Autodesk Inventor part; units mm, degrees
ref_plane "YZ Plane" through (0, 0, 0) normal (1, 0, 0) x (0, 1, 0)
ref_plane "XZ Plane" through (0, 0, 0) normal (0, 1, 0) x (-1, 0, 0)
ref_plane "XY Plane" through (0, 0, 0) normal (0, 0, 1) x (1, 0, 0)
sketch "Sketch1" plane through (0, 0, 0) normal (0, 1, 0) x (-1, 0, 0)
  line L0 (0, 0) -> (40.5, 0)
  line L1 (40.5, 0) -> (40.5, -20)
  line L2 (40.5, -20) -> (0, -20)
  line L3 (0, -20) -> (0, 0)
  dimension "d0" = 20
  dimension "d1" = 40.5
extrude "Extrusion1" add sketch "Sketch1" along normal blind 28
sketch "Sketch2" plane through (0, 28, 0) normal (0, 1, 0) x (1, 0, 0)
  line L0 (7.25, 0) -> (-47.75, 0)
  line L1 (-47.75, 0) -> (-47.75, 20)
  line L2 (-47.75, 20) -> (7.25, 20)
  line L3 (7.25, 20) -> (7.25, 0)
  line L4 (0, 20) -> (-40.5, 20)
  line L5 (-40.5, 20) -> (-40.5, 0)
  line L6 (-40.5, 0) -> (0, 0)
  dimension "d4" = 0
  dimension "d5" = 55
  dimension "d6" = 7.25
  dimension "d7" = 0
extrude "Extrusion2" add sketch "Sketch2" along normal blind 3.5
sketch "Sketch3" plane through (0, 31.5, 0) normal (0, 1, 0) x (1, 0, 0)
  circle A0 centre (-44.75, 5) radius 2.5
  circle A1 centre (-44.75, 15) radius 2.5
  line L0 (-47.75, 0) -> (7.25, 0)
  line L1 (7.25, 20) -> (-47.75, 20)
  line L2 (-47.75, 20) -> (-47.75, 0)
  point P0 (0, 0)
  dimension "d10" = 5
  dimension "d11" = 5
  dimension "d12" = 5
  dimension "d14" = 5
  dimension "d15" = 3
  dimension "d16" = 3
extrude "Extrusion3" cut sketch "Sketch3" against normal blind 3.5
ref_plane "Work Plane1" through (-20.25, 28, 0) normal (1, 0, 0) x (0, 0, -1)
mirror "Mirror1" about plane through (-20.25, 28, 0) normal (1, 0, 0) of "Extrusion3"
sketch "Sketch4" plane through (0, 31.5, 0) normal (0, 1, 0) x (1, 0, 0)
  line L0 (0, 0) -> (-40.5, 0)
  line L1 (-40.5, 0) -> (-40.5, 20)
  line L2 (-40.5, 20) -> (0, 20)
  line L3 (0, 20) -> (0, 0)
extrude "Extrusion4" add sketch "Sketch4" along normal blind 10
sketch "Sketch5" plane through (0, 41.5, 0) normal (0, 1, 0) x (1, 0, 0)
  circle A0 centre (-9, 10) radius 2.75
  line L0 (0, 0) -> (0, 20)
  line L1 (-40.5, 0) -> (0, 0)
  line L2 (-40.5, 20) -> (-40.5, 0)
  dimension "d22" = 10
  dimension "d23" = 5.5
  dimension "d40" = 31.5
extrude "Extrusion5" add sketch "Sketch5" along normal blind 6.5
sketch "Sketch6" plane through (0, 0, 0) normal (1, 0, 0) x (0, 0, -1)
  line L0 (6.75, 3) -> (13.25, 3)
  line L1 (13.25, 3) -> (13.25, 6.5)
  line L2 (13.25, 6.5) -> (6.75, 6.5)
  line L3 (6.75, 6.5) -> (6.75, 3)
  line L4 (0, 0) -> (20, 0)
  line L5 (0, 0) -> (0, 28)
  dimension "d26" = 3
  dimension "d27" = 6.5
  dimension "d28" = 3.5
  dimension "d29" = 6.75
extrude "Extrusion6" add sketch "Sketch6" along normal blind 6
sketch "Sketch7" plane through (6, 0, 0) normal (1, 0, 0) x (0, 0, -1)
  circle A0 centre (11.75, 4.75) radius 1.5
  circle A1 centre (8.25, 4.75) radius 1.5
  line L0 (6.75, 6.5) -> (6.75, 3)
  line L1 (13.25, 3) -> (13.25, 6.5)
  line L2 (6.75, 3) -> (13.25, 3)
  point P0 (0, 0)
  dimension "d32" = 3
  dimension "d33" = 3
  dimension "d34" = 1.5
  dimension "d35" = 1.5
  dimension "d36" = 1.75
  dimension "d37" = 1.75
extrude "Extrusion7" add sketch "Sketch7" along normal blind 30
equation "\"d33\" = d32"
equation "\"d37\" = d36"
properties part number "motor_25kg"
Input: part model. Units: mm. Frame: model coordinates. A direction names the side the tool comes from. Give positions to 0.01 mm unless a question says otherwise; leave off trailing zeros. Write each loop counter-clockwise with the first axis right and the second up, starting at its lowest first coordinate (ties: lowest second). Pieces come first, ordered by that corner, then holes. Notation, with made-up numbers: (-16.5, -15.75) -> (32.5, -15.75) arc R5 ccw to (32.5, -10.75) -> close; hole circle Ø9 at (-5.5, -2). An arc over 180 degrees is marked (long way). Use one line per item in the form item = value. Start each with the question number.
1) Ray query, probe 1 along X at (y, z) = (29, -15); probe 2 along Z at (x, y) = (4, 29); probe 3 along X at (y, z) = (7, -8.5). Return the intervals inside material, ascending. Write a range as from..to.
2) Section query B-B on z = -5. Return the cut outline in (x, y), then the cut area to 3 significant figures.
3) Draft query along Z for faces 4 (the flat face through (6, 5, -10)), 5 (the flat face through (-21, 20, -20)), 6 (the cylindrical face through (-6.46, 44.7, -11.05)). Return one class per face: pulls with the +Z half, pulls with the -Z half, needs draft (parallel to the pull), parting line crosses it, or undercut.
4) Section query C-C on y = 30. Return the cut outline in (x, z), then the cut area to 3 significant figures.
5) Pin query (flat end, axial travel): pin 1 (3 mm diameter, centred on x = 2, z = -8.5, fed in from -Y); pin 2 (5 mm diameter, centred on y = 12, z = -12.5, fed in from -X); pin 3 (1.8 mm diameter, centred on y = 30, z = -8, fed in from +X); pin 4 (3 mm diameter, centred on x = 4.25, z = -5, fed in from -Y). Return the tip coordinate at first contact, or that it passes through.
6) Section query D-D on x = -9. Return the cut outline in (y, z).
7) Set-up query: faces 1 (the flat face through (3, 3, -10)), 2 (the cylindrical face through (1.865, 29.774, -4.249)), 3 (the flat face through (3, 5, -13.25)). Return all of +Z, -Z, +X, -X, +Y, -Y with unobstructed straight access to the full face (end or side cutting, diameter ignored); none if empty.
8) Section query A-A on x = 4.25. Return the cut outline in (y, z).
Outcome:
q1.probe_1 = -47.75..-47.25, -42.25..1.75, 6.75..7.25
q1.probe_2 = -20..-17.49, -12.51..-7.49, -2.51..0
q1.probe_3 = -40.5..0
q2.outline = (-47.75, 28) -> (-47.25, 28) -> (-47.25, 31.5) -> (-47.75, 31.5) -> close; (-42.25, 28) -> (-40.5, 28) -> (-40.5, 0) -> (0, 0) -> (0, 28) -> (1.75, 28) -> (1.75, 31.5) -> (0, 31.5) -> (0, 41.5) -> (-40.5, 41.5) -> (-40.5, 31.5) -> (-42.25, 31.5) -> close; (6.75, 28) -> (7.25, 28) -> (7.25, 31.5) -> (6.75, 31.5) -> close
q2.area = 1,700 mm^2
q3.face_4 = undercut
q3.face_5 = pulls with the -Z half
q3.face_6 = parting line crosses it
q4.outline = (-47.75, -20) -> (7.25, -20) -> (7.25, 0) -> (-47.75, 0) -> close; hole circle Ø5 at (-44.75, -15); hole circle Ø5 at (-44.75, -5); hole circle Ø5 at (4.25, -15); hole circle Ø5 at (4.25, -5)
q4.area = 1,020 mm^2
q5.pin_1 = 3
q5.pin_2 = -40.5
q5.pin_3 = 7.25
q5.pin_4 = through
q6.outline = (0, -20) -> (41.5, -20) -> (41.5, -12.75) -> (48, -12.75) -> (48, -7.25) -> (41.5, -7.25) -> (41.5, 0) -> (0, 0) -> close
q7.face_1 = +Z, -Z, +X, -Y
q7.face_2 = +Y
q7.face_3 = -Z, +X, -Y
q8.outline = (3, -13.25) -> (6.5, -13.25) -> (6.5, -6.75) -> (3, -6.75) -> close; (28, -20) -> (31.5, -20) -> (31.5, -17.5) -> (28, -17.5) -> close; (28, -12.5) -> (31.5, -12.5) -> (31.5, -7.5) -> (28, -7.5) -> close; (28, -2.5) -> (31.5, -2.5) -> (31.5, 0) -> (28, 0) -> close
